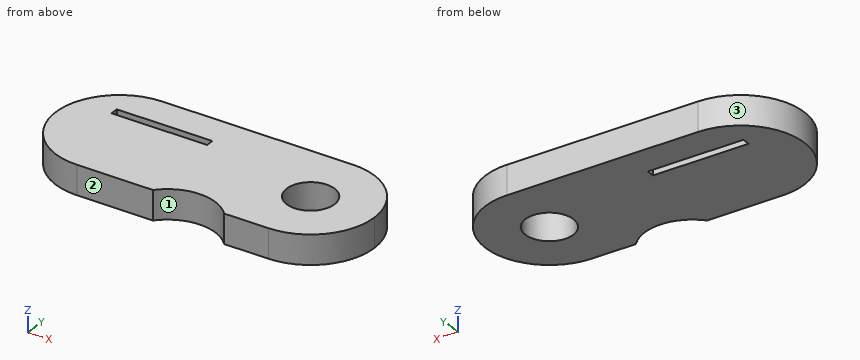
```python
from build123d import *

# Parameters (mm, degrees)
F1_DEPTH = 5.842
F2_R     = 4.7625
F3_DEPTH = 25.4
F4_W     = 19.05
F4_H     = 1.5875
F5_DEPTH = 25.4
F7_DEPTH = 25.4


# Not quite as in the source:
# - a feature names something its author has since deleted; it is built from what else it names


with BuildPart() as f1:
    # F0 (on Top) → F1 (new body)
    with BuildSketch(Plane.XY):
        with BuildLine():
            Line((-38.1, 25.4), (-38.1, 0))
            ThreePointArc((-38.1, 0), (-29.1197438789, 3.7197438789), (-25.4, 12.7))
            ThreePointArc((-25.4, 12.7), (-29.1197438789, 21.6802561211), (-38.1, 25.4))
        make_face()
        with BuildLine():
            ThreePointArc((0, 25.4), (-12.7, 12.7), (0, 0))
            Line((0, 0), (0, 25.4))
        make_face()
        with BuildLine():
            Line((-38.1, 0), (0, 0))
            ThreePointArc((0, 0), (-12.7, 12.7), (0, 25.4))
            Line((0, 25.4), (-38.1, 25.4))
            ThreePointArc((-38.1, 25.4), (-29.1197438789, 21.6802561211), (-25.4, 12.7))
            ThreePointArc((-25.4, 12.7), (-29.1197438789, 3.7197438789), (-38.1, 0))
        make_face()
        with BuildLine():
            Line((0, 25.4), (0, 0))
            ThreePointArc((0, 0), (8.9802561211, 3.7197438789), (12.7, 12.7))
            ThreePointArc((12.7, 12.7), (8.9802561211, 21.6802561211), (0, 25.4))
        make_face()
        with BuildLine():
            ThreePointArc((-38.1, 25.4), (-50.8, 12.7), (-38.1, 0))
            Line((-38.1, 0), (-38.1, 25.4))
        make_face()
    extrude(amount=F1_DEPTH)

    # F2 (on face) → F3 (cut)
    with BuildSketch(Plane.XY.offset(5.842)):
        with Locations((0, 12.7)):
            Circle(F2_R)
    extrude(amount=-F3_DEPTH, mode=Mode.SUBTRACT)

    # F4 (on face) → F5 (cut)
    with BuildSketch(Plane.XY.offset(5.842)):
        with Locations((-33.3375, 18.25625)):
            Rectangle(F4_W, F4_H)
    extrude(amount=-F5_DEPTH, mode=Mode.SUBTRACT)

    # F6 (on face) → F7 (cut)
    with BuildSketch(Plane(origin=(0, 0, 0), x_dir=(1, 0, 0), z_dir=(0, 0, -1))):
        with BuildLine():
            Line((-8.7754841714, 0), (-22.9745158286, 0))
            ThreePointArc((-22.9745158286, 0), (-15.875, -3.175), (-8.7754841714, 0))
        make_face()
    extrude(amount=-F7_DEPTH, mode=Mode.SUBTRACT)


solid = f1.part
```
The listing builds one solid part. Answer for the finished solid, in the listing's coordinates (mm). Face numbers are marked on the shaded views. Give positions to 0.01 mm unless a question says otherwise; leave off trailing zeros. Order: outer loops, then holes, each group sorted by start corner. A loop starts at its lowest first (then second) coordinate and runs counter-clockwise, first axis right, second up. Notation, with made-up numbers: (51.25, 38) -> (110.25, 38) arc R24 cw to (110.25, 69) -> close; hole circle Ø5 at (60.5, 11.25). An arc over 180 degrees is marked (long way). One line per item, written item: value.
1) Find section A-A, the plane x = -30.5. Determine the outline of the cut face in (y, z).
Reported:
outline: (0, 0) -> (17.46, 0) -> (17.46, 5.84) -> (0, 5.84) -> close; (19.05, 0) -> (25.4, 0) -> (25.4, 5.84) -> (19.05, 5.84) -> close
2) Find the intervals of material crossed by line 1 (Y direction, x = 0, z = 2.7); line 2 (X direction, y = 15.5, z = 4.4); line 3 (Y direction, x = -26, z = 2.5), in increasing order.
Reported:
line 1: y = 0 to 7.94, 17.46 to 25.4
line 2: x = -50.49 to -3.85, 3.85 to 12.39
line 3: y = 0 to 17.46, 19.05 to 25.4
3) Find section C-C, the plane z = 1.1. Count the separate pieces of the cut face and the enclosed holes in it, plus the area to 3 significant figures.
Reported:
separate pieces: 1
enclosed holes: 2
area: 1,340 mm^2
4) Flat-ended cylindrical pins translate along their axes: P1, Ø0.5, axis at y = 18, z = 2, coming from the +X side; P2, Ø0.5, axis at y = 18, z = 2.5, coming from the -X side; P3, Ø1.5, axis at y = 8, z = 3.5, coming from the +X side; P4, Ø7.5, axis at x = 0, y = 12.7, coming from the +Z side. Find the tip coordinate at first contact, or state that the pin passes through.
Reported:
P1: stops at x = 11.65
P2: stops at x = -49.75
P3: stops at x = 12.07
P4: passes through
5) Find section B-B, the plane y = 16. Determine the outline of the cut face in (x, z), plus the area to 3 significant figures.
Reported:
outline: (-50.36, 0) -> (-3.43, 0) -> (-3.43, 5.84) -> (-50.36, 5.84) -> close; (3.43, 0) -> (12.26, 0) -> (12.26, 5.84) -> (3.43, 5.84) -> close
area: 326 mm^2
6) Determine the mould class of the marked faces 1, 2 and 3 for opening direction X: pulls with the +X half, pulls with the -X half, needs draft (parallel to the pull), parting line crosses it, or undercut.
Reported:
face 1: undercut
face 2: needs draft
face 3: pulls with the -X half
7) Find section D-D, the plane y = 3.75. Determine the outline of the cut face in (x, z), plus the area to 3 significant figures.
Reported:
outline: (-47.11, 0) -> (9.01, 0) -> (9.01, 5.84) -> (-47.11, 5.84) -> close
area: 328 mm^2
